Part print with two shaded views. Sizes in mm from the minimum x, y, z corner. Round coordinates to 2 decimals unless told otherwise and drop trailing zeros. Order: outer loops, then holes, each group sorted by start corner. A loop starts at its lowest first (then second) coordinate and runs counter-clockwise, first axis right, second up. Notation, with made-up numbers: M 10,61 L 58,61 A21 cw 58,97 Z; hole C -32,20.5 d9. An arc over 180 degrees is marked long. One line per question, with ' | ' between items.
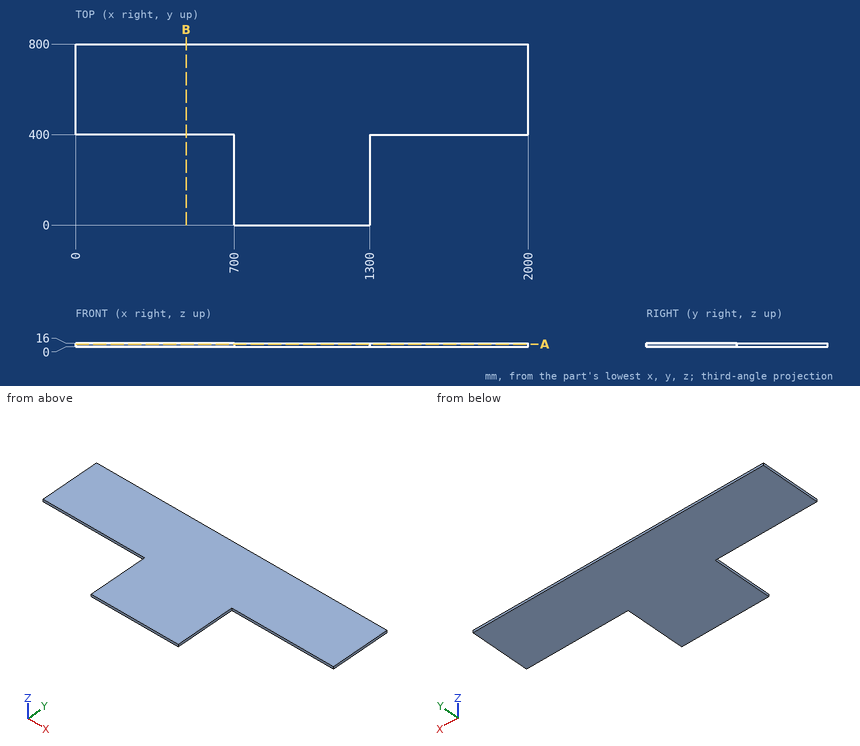
1) Probe line 1 (Y direction, x = 1807.5, z = 6.25); line 2 (X direction, y = 140, z = 13.5). List the from-to ranges inside material, lowest first. Write a range as [from, to].
The answers:
line 1: y = [400, 800] | line 2: x = [700, 1300]
2) Saw through at A-A (z = 11.5). List the corners of the cut face in (x, y), plus the area to 3 significant figures.
The answers:
outline: M 0,400 L 700,400 L 700,0 L 1300,0 L 1300,400 L 2000,400 L 2000,800 L 0,800 Z | area: 1,040,000 mm²
3) Saw through at B-B (x = 489). List the corners of the cut face in (y, z), plus the area to 3 significant figures.
The answers:
outline: M 400,0 L 800,0 L 800,16 L 400,16 Z | area: 6,400 mm²
4) Drop flat-ended pins along their axis: pin 1 (1.5 mm diameter, centred on x = 380.5, z = 3, fed in from -Y); pin 2 (2 mm diameter, centred on y = 338.5, z = 7.5, fed in from -X). Give the stop position or say it passes through.
The answers:
pin 1: stops at y = 400 | pin 2: stops at x = 700
